Design review of the part built by this model. Coordinates are the model's own, in mm. Face numbers are marked on the shaded views. A direction names the side the tool comes from. Give positions to 0.01 mm unless a question says otherwise; leave off trailing zeros. Loops run counter-clockwise (first coordinate to the right, second up) from the corner with the lowest first, then second, coordinate; pieces in that order, holes last.
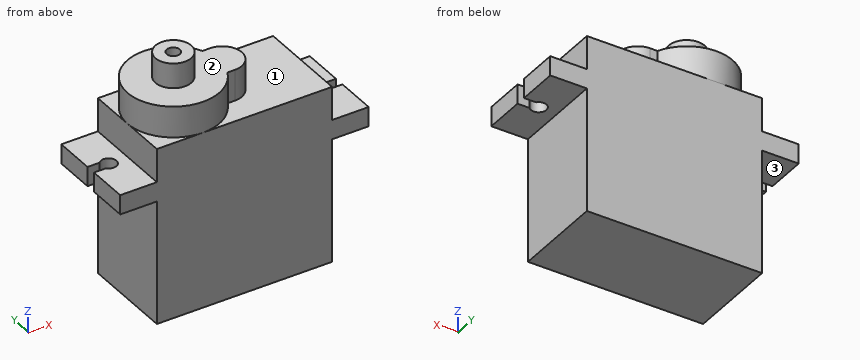
from build123d import *

# Parameters (mm, degrees)
F1_DEPTH  = 11.8
F3_DEPTH  = 4
F5_DEPTH  = 25
F7_DEPTH  = 25
F8_R      = 2.3
F9_DEPTH  = 3.2
F10_R     = 0.85
F11_DEPTH = 1.7


with BuildPart() as f1:
    # F0 (on Front) → F1 (new body)
    with BuildSketch(Plane.XZ):
        Polygon((0, 15.9), (0, 0), (22.5, 0), (22.5, 15.9), (27.2, 15.9), (27.2, 18.4), (22.5, 18.4), (22.5, 22.7), (0, 22.7), (0, 18.4), (-4.7, 18.4), (-4.7, 15.9), align=None)
    extrude(amount=-F1_DEPTH)

    # F2 (on face) → F3 (join)
    with BuildSketch(Plane.XY.offset(22.7)):
        with BuildLine():
            Line((12.2, 8.4), (11.244156, 8.4))
            ThreePointArc((11.244156, 8.4), (0, 5.9), (11.244156, 3.4))
            Line((11.244156, 3.4), (12.2, 3.4))
            ThreePointArc((12.2, 3.4), (14.7, 5.9), (12.2, 8.4))
        make_face()
    extrude(amount=F3_DEPTH)

    # F4 (on face) → F5 (cut)
    with BuildSketch(Plane.XY.offset(18.4)):
        with BuildLine():
            Line((27.2, 5.25), (27.2, 6.55))
            Line((27.2, 6.55), (25.659934, 6.55))
            ThreePointArc((25.659934, 6.55), (23.9, 5.9), (25.659934, 5.25))
            Line((25.659934, 5.25), (27.2, 5.25))
        make_face()
    extrude(amount=-F5_DEPTH, mode=Mode.SUBTRACT)

    # F6 (on face) → F7 (cut)
    with BuildSketch(Plane.XY.offset(18.4)):
        with BuildLine():
            Line((-3.159934, 6.55), (-4.7, 6.55))
            Line((-4.7, 6.55), (-4.7, 5.25))
            Line((-4.7, 5.25), (-3.159934, 5.25))
            ThreePointArc((-3.159934, 5.25), (-1.4, 5.9), (-3.159934, 6.55))
        make_face()
    extrude(amount=-F7_DEPTH, mode=Mode.SUBTRACT)

    # F8 (on face) → F9 (join)
    with BuildSketch(Plane.XY.offset(26.7)):
        with Locations((5.9, 5.9)):
            Circle(F8_R)
    extrude(amount=F9_DEPTH)

    # F10 (on face) → F11 (cut)
    with BuildSketch(Plane.XY.offset(29.9)):
        with Locations((5.9, 5.9)):
            Circle(F10_R)
    extrude(amount=-F11_DEPTH, mode=Mode.SUBTRACT)


solid = f1.part
Q1. Take a section at B-B (x = 3). Give the boundary of the cut face in (y, z).
Results:
outline: (0, 0) - (11.8, 0) - (11.8, 22.7) - (11.04, 22.7) - (11.04, 26.7) - (0.76, 26.7) - (0.76, 22.7) - (0, 22.7) - close
Q2. Take a section at D-D (z = 24.5). Give the boundary of the cut face in (x, y), plus the area to 3 significant figures.
Results:
outline: (11.24, 3.4) - (12.2, 3.4) arc R2.5 ccw to (12.2, 8.4) - (11.24, 8.4) arc R5.9 ccw (long way) to start
area: 122 mm2
Q3. Insertion check: pin 1 (1.5 mm diameter, centred on x = -1.5, z = 19.5, fed in from -Y); pin 2 (2 mm diameter, centred on y = 5, z = 21.5, fed in from -X); pin 3 (5 mm diameter, centred on x = -2, y = 4.5, fed in from +Z). Each pin has a flat end and moves straight along its axis. Give the tip position at first contact, or say it passes through.
Results:
pin 1: passes through
pin 2: stops at x = 0
pin 3: stops at z = 26.7
Q4. Take a section at A-A (x = 24.9). Give the boundary of the cut face in (y, z).
Results:
outline: (0, 15.9) - (4.9, 15.9) - (4.9, 18.4) - (0, 18.4) - close; (6.9, 15.9) - (11.8, 15.9) - (11.8, 18.4) - (6.9, 18.4) - close
Q5. Take a section at C-C (y = 9). Give the boundary of the cut face in (x, z).
Results:
outline: (-4.7, 15.9) - (0, 15.9) - (0, 0) - (22.5, 0) - (22.5, 15.9) - (27.2, 15.9) - (27.2, 18.4) - (22.5, 18.4) - (22.5, 22.7) - (10.92, 22.7) - (10.92, 26.7) - (0.88, 26.7) - (0.88, 22.7) - (0, 22.7) - (0, 18.4) - (-4.7, 18.4) - close
Q6. Wall thickness on line 1 (Y direction, x = 24.9, z = 17.35); line 2 (Y direction, x = 5.9, z = 29.4); line 3 (Z direction, x = 3.5, y = 10.75): over which ranges is each line inside the solid? List them lowest first.
Results:
line 1: y = 0 to 4.9, 6.9 to 11.8
line 2: y = 3.6 to 5.05, 6.75 to 8.2
line 3: z = 0 to 26.7
Q7. Tool access review of the marked faces 1, 2 and 3: name each direction out of +Z, -Z, +X, -X, +Y, -Y from which nothing blocks a thin tool from reaching the whole face with its end or side.
Results:
face 1: +Z, +X
face 2: +Z
face 3: -Z, -X, +Y, -Y
